from build123d import *


with BuildPart() as part:
    # Sketch1 → Revolve-Thin1 (revolve)
    with BuildSketch(Plane(origin=(-3.343067137, 93.173104477, 24.269036423), x_dir=(1, 0, 0), z_dir=(0, 0, 1)), mode=Mode.PRIVATE) as revolve_thin1_sk:
        Polygon((-33.656932863, 68.327933214), (-33.656932863, 62.327933214), (-35.656932863, 62.327933214), (-35.656932863, 60.327933214), (-33.656932863, 60.327933214), (-33.656932863, 58.327933214), (-41.656932863, 50.327933214), (-41.656932863, -89.672066786), (-33.656932863, -95.273727092), (-28.656932863, -95.273727092), (-25.656932863, -93.173104477), (3.343067137, -93.173104477), (3.343067137, -94.173104477), (-25.341634074, -94.173104477), (-28.341634074, -96.273727092), (-33.972231651, -96.273727092), (-42.656932863, -90.192633837), (-42.656932863, 50.742146776), (-34.656932863, 58.742146776), (-34.656932863, 59.327933214), (-36.656932863, 59.327933214), (-36.656932863, 63.327933214), (-34.656932863, 63.327933214), (-34.656932863, 68.327933214), align=None)
    revolve(revolve_thin1_sk.sketch.rotate(Axis((0, 0, 24.269036423), (0, 1, 0)), 270), axis=Axis((0, 0, 24.269036423), (0, 1, 0)))


solid = part.part
Can you work these out from the model? Positions are in its coordinate system, mm. A direction names the side the tool comes from. Coordinates: 2 decimals unless noted, no trailing zeros. Write each loop counter-clockwise with the first axis right and the second up, starting at its lowest first coordinate (ties: lowest second). Pieces come first, ordered by that corner, then holes. Notation, with made-up numbers: M 74.5,69 L 122.5,69 A15 cw 122.5,82 Z; hole C -36,-36 d8. An arc over 180 degrees is marked long. Use one line per item in the form item = value.
Q1. If we section it at A-A (y = 132): Write out the boundary of the cut face in (x, z), then the cut area to 3 significant figures.
Model answer:
outline = C 0,24.27 d92; hole C 0,24.27 d90
area = 286 mm^2
Q2. We'd pull the mould along X, two halves only. Please class faces 5 (the flat face through (8.3, 161.501, -12.1)), 6 (the cylindrical face through (23.122, 152.212, 54.425)), 7 (the flat face through (23, 155.501, -5)): +X half, -X half, draft (parallel to the pull), parting line (faces both ways), or undercut.
Model answer:
face_5 = draft
face_6 = parting line
face_7 = undercut
Q3. For faces 1 (the cylindrical face through (14.17, 158.46, -9.91)), 2 (the flat face through (0, -1, 24)), 3 (the flat face through (27.5, -3.101, 7.5)), 4 (the flat face through (-29, 153.501, 1)), which set-ups out of +Z, -Z, +X, -X, +Y, -Y let a thin tool reach every point of the face, with its end or its side?
Model answer:
face_1 = +Y
face_2 = -Y
face_3 = +Z, -Z, +X, -X, -Y
face_4 = none
Q4. For P1, Ø2, axis at y = 111.5, z = 39, coming from the -X side; P2, Ø8, axis at x = -20, y = 145, coming from the +Z side; P3, Ø8, axis at y = 55, z = 19, coming from the -X side, each with a flat end and sliding along its axis, tell me the tip position at first contact or that it passes through.
Model answer:
P1 = -43.9
P2 = 67.34
P3 = -45.98
Q5. I need wall thicknesses on line 1 along Y through (x, z) = (1, 51); line 2 along X through (y, z) = (96, 47.5); line 3 along X through (y, z) = (53, -7). Which ranges of each line are inside material? Lowest first, please. Write a range as from..to.
Model answer:
line_1 = -1..0
line_2 = -39.7..-38.54, 38.54..39.7
line_3 = -33.74..-32.36, 32.36..33.74
